```python
from build123d import *

# Parameters (mm, degrees)
SKETCH_1_R          = 22
EXTRUDE_1_DEPTH     = 3
SKETCH_6_R          = 24
CUT_EXTRUDE_1_DEPTH = 0.1
SKETCH_7_W          = 161.718450326
SKETCH_7_H          = 100.382420291
CUT_EXTRUDE_2_DEPTH = 0.1
SKETCH_8_W          = 2
SKETCH_8_H          = 101.647080703
CUT_EXTRUDE_3_DEPTH = 0.1
SKETCH_9_W          = 185.430833072
SKETCH_9_H          = 2
CUT_EXTRUDE_4_DEPTH = 0.1


with BuildPart() as part:
    # Эскиз1 → Бобышка-Вытянуть1 (new body)
    with BuildSketch(Plane.XY):
        with BuildLine():
            Line((-74, 53), (74, 53))
            ThreePointArc((74, 53), (74.707106781, 52.707106781), (75, 52))
            Line((75, 52), (75, -36))
            ThreePointArc((75, -36), (74.707106781, -36.707106781), (74, -37))
            Line((74, -37), (-74, -37))
            ThreePointArc((-74, -37), (-74.707106781, -36.707106781), (-75, -36))
            Line((-75, -36), (-75, 52))
            ThreePointArc((-75, 52), (-74.707106781, 52.707106781), (-74, 53))
        make_face()
        Circle(SKETCH_1_R, mode=Mode.SUBTRACT)
    extrude(amount=EXTRUDE_1_DEPTH)

    # Эскиз6 → Вырез-Вытянуть1 (cut)
    with BuildSketch(Plane.XY.offset(3)):
        Circle(SKETCH_6_R)
    extrude(amount=-CUT_EXTRUDE_1_DEPTH, mode=Mode.SUBTRACT)

    # Эскиз7 → Вырез-Вытянуть2 (cut)
    with BuildSketch(Plane.XY.offset(3)):
        with Locations((0.395206379, 8.158082552)):
            Rectangle(SKETCH_7_W, SKETCH_7_H)
        with BuildLine():
            Line((72, 51), (-72, 51))
            ThreePointArc((-72, 51), (-72.707106781, 50.707106781), (-73, 50))
            Line((-73, 50), (-73, -34))
            ThreePointArc((-73, -34), (-72.707106781, -34.707106781), (-72, -35))
            Line((-72, -35), (72, -35))
            ThreePointArc((72, -35), (72.707106781, -34.707106781), (73, -34))
            Line((73, -34), (73, 50))
            ThreePointArc((73, 50), (72.707106781, 50.707106781), (72, 51))
        make_face(mode=Mode.SUBTRACT)
    extrude(amount=-CUT_EXTRUDE_2_DEPTH, mode=Mode.SUBTRACT)

    # Эскиз8 → Вырез-Вытянуть3 (cut)
    with BuildSketch(Plane.XY.offset(3)):
        with Locations((0, 5.154514071)):
            Rectangle(SKETCH_8_W, SKETCH_8_H)
    extrude(amount=-CUT_EXTRUDE_3_DEPTH, mode=Mode.SUBTRACT)

    # Эскиз9 → Вырез-Вытянуть4 (cut)
    with BuildSketch(Plane.XY.offset(3)):
        with Locations((6.718508445, 0)):
            Rectangle(SKETCH_9_W, SKETCH_9_H)
    extrude(amount=-CUT_EXTRUDE_4_DEPTH, mode=Mode.SUBTRACT)


solid = part.part
```
Could you check a few things on this model? Use its own coordinates, in mm. Round coordinates to 2 decimals unless told otherwise and drop trailing zeros. Loops run counter-clockwise (first coordinate to the right, second up) from the corner with the lowest first, then second, coordinate; pieces in that order, holes last.
Q1. I want a section at A-A (z = 0.7). Write out the boundary of the cut face in (x, y), and give its area (3 significant figures).
Q2. Thinking about a two-plate mould opening in Y: for faces 1 (the flat face through (75, 9, 1)), 2 (the flat face through (-1, 53, 1)), 3 (the cylindrical face through (-4.769, -21.477, 1.43)), which applies, pulls with the +Y half, pulls with the -Y half, needs draft (parallel to the pull), parting line crosses it, or undercut?
Q3. Please list where these lines run through material, in increasing order: L1, parallel to Y at x = 0, z = 1.85; L2, parallel to X at y = 0, z = 2; L3, parallel to Y at x = 15, z = 0.85.
Q4. I want a section at B-B (y = -11.5). Write out the boundary of the cut face in (x, z) (3 decimals), and give its area (3 significant figures).
Q5. I want a section at C-C (x = 15). Write out the boundary of the cut face in (y, z) (3 decimals), and give its area (3 significant figures).
Answer below:
1. outline: (-75, -36) arc R1 ccw to (-74, -37) - (74, -37) arc R1 ccw to (75, -36) - (75, 52) arc R1 ccw to (74, 53) - (-74, 53) arc R1 ccw to (-75, 52) - close; hole circle Ø44 at (0, 0)
1. area: 12,000 mm2
2. face 1: needs draft
2. face 2: pulls with the +Y half
2. face 3: undercut
3. L1: y = -37 to -22, 22 to 53
3. L2: x = -75 to -22, 22 to 75
3. L3: y = -37 to -16.09, 16.09 to 53
4. outline: (-75, 0) - (-18.755, 0) - (-18.755, 2.9) - (-21.065, 2.9) - (-21.065, 3) - (-73, 3) - (-73, 2.9) - (-75, 2.9) - close; (18.755, 0) - (75, 0) - (75, 2.9) - (73, 2.9) - (73, 3) - (21.065, 3) - (21.065, 2.9) - (18.755, 2.9) - close
4. area: 337 mm2
5. outline: (-37, 0) - (-16.093, 0) - (-16.093, 2.9) - (-18.735, 2.9) - (-18.735, 3) - (-35, 3) - (-35, 2.9) - (-37, 2.9) - close; (16.093, 0) - (53, 0) - (53, 2.9) - (51, 2.9) - (51, 3) - (18.735, 3) - (18.735, 2.9) - (16.093, 2.9) - close
5. area: 173 mm2
